```python
from build123d import *

# Parameters (mm, degrees)
ESQUISSE1_R           = 10
ESQUISSE1_R_2         = 5
BOSS_EXTRU_1_DEPTH    = 15
TROU_TARAUD_M31_D     = 2.5
TROU_TARAUD_M31_DEPTH = 8.5
TROU_TARAUD_M31_TIP   = 0.751075774
TROU_TARAUD_M32_D     = 2.5
TROU_TARAUD_M32_DEPTH = 8.5
TROU_TARAUD_M32_TIP   = 0.751075774


with BuildPart() as part:
    # Esquisse1 → Boss.-Extru.1 (new body)
    with BuildSketch(Plane.XY):
        Circle(ESQUISSE1_R)
        Circle(ESQUISSE1_R_2, mode=Mode.SUBTRACT)
    extrude(amount=BOSS_EXTRU_1_DEPTH)

    # Trou taraudé M31
    with Locations(Plane(origin=(10, 0, 0), x_dir=(0, 0, -1), z_dir=(1, 0, 0))):
        with Locations((-7.5, 0)):
            Hole(TROU_TARAUD_M31_D / 2, depth=TROU_TARAUD_M31_DEPTH)
            with Locations((0, 0, -(TROU_TARAUD_M31_DEPTH + TROU_TARAUD_M31_TIP / 2))):  # 118° drill point
                Cone(0, TROU_TARAUD_M31_D / 2, TROU_TARAUD_M31_TIP, mode=Mode.SUBTRACT)

    # Trou taraudé M32
    with Locations(Plane(origin=(-10, 0, 0), x_dir=(0, 0, -1), z_dir=(-1, 0, 0))):
        with Locations((-7.5, 0)):
            Hole(TROU_TARAUD_M32_D / 2, depth=TROU_TARAUD_M32_DEPTH)
            with Locations((0, 0, -(TROU_TARAUD_M32_DEPTH + TROU_TARAUD_M32_TIP / 2))):  # 118° drill point
                Cone(0, TROU_TARAUD_M32_D / 2, TROU_TARAUD_M32_TIP, mode=Mode.SUBTRACT)


solid = part.part
```
Geometry check sheet. Reference: the model listing, model coordinates, mm. Coordinates: 2 decimals unless noted, no trailing zeros. Order: outer loops, then holes, each group sorted by start corner. A loop starts at its lowest first (then second) coordinate and runs counter-clockwise, first axis right, second up. Notation, with made-up numbers: M 52.5,29 L 92.5,29 A10 ccw 92.5,33 Z; hole C 49,32.25 d2. An arc over 180 degrees is marked long. One line per question, with ' | ' between items. Start each with the question number.
Item 1: Cross-section at A-A on x = 0. Enter the section's corners in (y, z).
Item 2: Material ranges on L1, parallel to Y at x = 0, z = 3.75; L2, parallel to Z at x = 5.5, y = 0; L3, parallel to X at y = -2, z = 1.75, recorded low to high. Write a range as [from, to].
Item 3: Cross-section at B-B on y = 0. Enter the section's corners in (x, z).
Item 4: Cross-section at C-C on y = 3.75. Enter the section's corners in (x, z).
Item 5: Gauge pin test, flat ends, axial feed: pin 1 (5 mm diameter, centred on x = -7, z = 8.5, fed in from -Y); pin 2 (1 mm diameter, centred on x = -2.5, z = 10.5, fed in from +Y). Record the tip position at first contact, or that the pin passes through.
Item 6: Cross-section at D-D on z = 13.25. Enter the section's corners in (x, y), then the cut area to 3 significant figures.
Item 7: Draft check along Y on faces 1 (the flat face through (-5, -2, 0)), 2 (the cylindrical face through (9.54, 3, 7.4)), 3 (the cylindrical face through (7.38, 0.05, 6.25)). Enter one of: pulls with the +Y half, pulls with the -Y half, needs draft (parallel to the pull), parting line crosses it, or undercut.
Findings:
1) outline: M -10,0 L -5,0 L -5,15 L -10,15 Z; M 5,0 L 10,0 L 10,15 L 5,15 Z
2) L1: y = [-10, -5], [5, 10] | L2: z = [0, 6.25], [8.75, 15] | L3: x = [-9.8, -4.58], [4.58, 9.8]
3) outline: M -10,0 L -5,0 L -5,6.25 L -10,6.25 Z; M -10,8.75 L -5,8.75 L -5,15 L -10,15 Z; M 5,0 L 10,0 L 10,6.25 L 5,6.25 Z; M 5,8.75 L 10,8.75 L 10,15 L 5,15 Z
4) outline: M -9.27,0 L -3.31,0 L -3.31,15 L -9.27,15 Z; M 3.31,0 L 9.27,0 L 9.27,15 L 3.31,15 Z
5) pin 1: stops at y = -8.93 | pin 2: stops at y = 9.8
6) outline: C 0,0 d20; hole C 0,0 d10 | area: 236 mm²
7) face 1: needs draft | face 2: parting line crosses it | face 3: undercut
